from build123d import *

# Parameters (mm, degrees)
F0_R     = 41.0268992287
F1_DEPTH = 101.6
F2_R     = 36.535273012
F3_DEPTH = 97.79
F4_R     = 1.5330256121
F6_W     = 19.5752624422
F6_H     = 75.4010118544
F8_W     = 26.9523151219
F8_H     = 60.3598859161
F9_DEPTH = 51.1780356548
F10_R    = 22.9953841816
F11_R    = 5.08
F12_R    = 5.08


with BuildPart() as f1:
    # F0 (on Top) → F1 (new body)
    with BuildSketch(Plane.XY):
        Circle(F0_R)
    extrude(amount=F1_DEPTH)

    # F2 (on face) → F3 (cut)
    with BuildSketch(Plane.XY.offset(101.6)):
        Circle(F2_R)
    extrude(amount=-F3_DEPTH, mode=Mode.SUBTRACT)

    # F4
    f4_edges = [f1.edges().sort_by_distance(p)[0] for p in [
        (-36.535273, 0, 101.6),
        (-41.026899, 0, 101.6),
    ]]
    fillet(f4_edges, radius=F4_R)

    # F6 (on offset) → F7 (join, up to the next surface of F1)
    with BuildSketch(Plane.XZ.offset(76.2)):
        with Locations((-0.362505205, 49.4942422956)):
            Rectangle(F6_W, F6_H)
    extrude(until=Until.NEXT, dir=(0, 1, 0))

    # F8 (on face) → F9 (cut, through all)
    with BuildSketch(Plane(origin=(-10.1501364261, 0, 0), x_dir=(0, -1, 0), z_dir=(-1, 0, 0))):
        with Locations((57.1689289063, 50.295223482)):
            Rectangle(F8_W, F8_H)
    extrude(amount=-F9_DEPTH, mode=Mode.SUBTRACT)

    # F10
    f10_edges = [f1.edges().sort_by_distance(p)[0] for p in [
        (-0.362505, -76.2, 87.194748),
        (-0.362505, -76.2, 11.793736),
        (-0.362505, -70.645086, 20.115281),
        (-0.362505, -70.645086, 80.475166),
    ]]
    fillet(f10_edges, radius=F10_R)

    # F11
    f11_edges = [f1.edges().sort_by_distance(p)[0] for p in [
        (-10.150136, -69.464808, 80.459556),
    ]]
    fillet(f11_edges, radius=F11_R)

    # F12
    f12_edges = [f1.edges().sort_by_distance(p)[0] for p in [
        (9.425126, -69.464808, 80.459556),
    ]]
    fillet(f12_edges, radius=F12_R)


solid = f1.part
Read the model definition and answer for the solid it produces. Units are mm, in the model's axes. A direction names the side the tool comes from. Round coordinates to 2 decimals unless told otherwise and drop trailing zeros. Write each loop counter-clockwise with the first axis right and the second up, starting at its lowest first coordinate (ties: lowest second). Pieces come first, ordered by that corner, then holes.
1. Determine the mould class of faces 1 (the face through (0, -43.693, 50)), 2 (the face through (7.898, -46.474, 13.242)), 3 (the face through (-0.297, -69.285, 18.351)) for opening direction Y: pulls with the +Y half, pulls with the -Y half, needs draft (parallel to the pull), parting line crosses it, or undercut.
2. The part is cut by section C-C, the plane z = 7.5. Determine the outline of the cut face in (x, y).
3. Straight lines are drawn through the part: L1, parallel to Y at x = 0, z = 57; L2, parallel to Y at x = 0, z = 67.5; L3, parallel to Y at x = -1.5, z = 97. For each, find the intervals that lie inside material, in ascending order.
4. The part is cut by section A-A, the plane x = 0. Determine the outline of the cut face in (y, z), then the cut area to 3 significant figures.
5. Given pin 1 Ø2 at (x, y) = (-3, -46.5) entering from -Z; pin 2 Ø16 at (x, z) = (-1.5, 52.5) entering from +Y; pin 3 Ø7.5 at (x, y) = (-1, -47.5) entering from +Z, each flat-ended and moving along its own axis, determine where each tip first touches the part or whether it passes through.
6. The part is cut by section D-D, the plane z = 31.5. State how many separate pieces and enclosed holes the cut face has, then the cut area to 3 significant figures.
7. Which of the six approach directions +Z, -Z, +X, -X, +Y, -Y give full straight-line access (tool end or side, diameter ignored) to faces 4 (the face through (0, -46, 80.475)), 5 (the face through (-8.62, -46.57, 85.75)), 6 (the face through (-8.62, -46.38, 13.24)), 7 (the face through (-10.15, -43, 49)), 8 (the face through (-4.756, 36.224, 52.612))?
8. The part is cut by section B-B, the plane y = 0. Determine the outline of the cut face in (x, z), then the cut area to 3 significant figures.
Values:
1. face 1: undercut
1. face 2: needs draft
1. face 3: pulls with the -Y half
2. outline: circle Ø82.05 at (0, 0); hole circle Ø73.07 at (0, 0)
3. L1: y = -76.2 to -70.65, -43.69 to -36.54, 36.54 to 41.03
3. L2: y = -75.96 to -68.35, -43.69 to -36.54, 36.54 to 41.03
3. L3: y = -41 to -36.5, 36.5 to 41
4. outline: (-76.2, 34.79) arc R23 ccw to (-53.2, 11.79) - (-41.03, 11.79) - (-41.03, 0) - (41.03, 0) - (41.03, 100.07) arc R1.53 ccw to (39.49, 101.6) - (38.07, 101.6) arc R1.53 ccw to (36.54, 100.07) - (36.54, 3.81) - (-36.54, 3.81) - (-36.54, 100.07) arc R1.53 ccw to (-38.07, 101.6) - (-39.49, 101.6) arc R1.53 ccw to (-41.03, 100.07) - (-41.03, 87.19) - (-53.2, 87.19) arc R23 ccw to (-76.2, 64.2) - close; hole (-70.65, 43.11) arc R23 ccw to (-47.65, 20.12) - (-43.69, 20.12) - (-43.69, 80.48) - (-47.65, 80.48) arc R23 ccw to (-70.65, 57.48) - close
4. area: 2,210 mm2
5. pin 1: stops at z = 11.79
5. pin 2: stops at y = 41.03
5. pin 3: stops at z = 87.19
6. separate pieces: 2
6. enclosed holes: 1
6. area: 1,310 mm2
7. face 4: +X, -X
7. face 5: +Z, -X, -Y
7. face 6: -Z, -X, -Y
7. face 7: +Z, -Z, -X, -Y
7. face 8: +Z
8. outline: (-41.03, 0) - (41.03, 0) - (41.03, 100.07) arc R1.53 ccw to (39.49, 101.6) - (38.07, 101.6) arc R1.53 ccw to (36.54, 100.07) - (36.54, 3.81) - (-36.54, 3.81) - (-36.54, 100.07) arc R1.53 ccw to (-38.07, 101.6) - (-39.49, 101.6) arc R1.53 ccw to (-41.03, 100.07) - close
8. area: 1,190 mm2
